from build123d import *

# Parameters (mm, degrees)
F0_W     = 80
F0_H     = 90
F1_DEPTH = 50
F2_T     = -2.5
F3_R     = 19.815
F4_DEPTH = 90.001


with BuildPart() as f1:
    # F0 (on Top) → F1 (new body)
    with BuildSketch(Plane.XY):
        Rectangle(F0_W, F0_H)
    extrude(amount=F1_DEPTH)

    # F2
    f2_openings = [f1.faces().sort_by_distance(p)[0] for p in [
        (0, 0, 50),
    ]]
    offset(amount=F2_T, openings=f2_openings)

    # F3 (on face) → F4 (cut, through all)
    with BuildSketch(Plane.XZ.offset(45)):
        with Locations((0, 25)):
            Circle(F3_R)
    extrude(amount=-F4_DEPTH, mode=Mode.SUBTRACT)


solid = f1.part
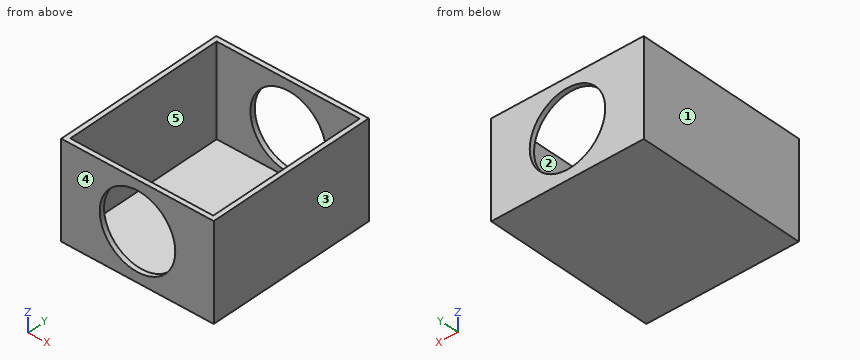
Source: CAD feature listing. Evaluate the final solid. Frame: model axes, mm. Face numbers are marked on the shaded views. A direction names the side the tool comes from. Round coordinates to 2 decimals unless told otherwise and drop trailing zeros. Loops run counter-clockwise (first coordinate to the right, second up) from the corner with the lowest first, then second, coordinate; pieces in that order, holes last. Notation, with made-up numbers: M 49,0.5 L 106,0.5 A15 ccw 106,25.5 Z; hole C 43.25,18.25 d11. An arc over 180 degrees is marked long. Return JSON: item names as keys, results as strings. Group by question number.
1. Section query C-C on y = 36.5. Output: boundary loops of the cut face in (x, z), and give its area (4 significant figures).
2. Section query A-A on x = 0. Output: boundary loops of the cut face in (y, z) (3 decimals).
3. Pin query (flat end, axial travel): pin 1 (1 mm diameter, centred on x = -25, y = -7.5, fed in from +Z); pin 2 (24 mm diameter, centred on x = 0, z = 25, fed in from -Y); pin 3 (3 mm diameter, centred on x = 12.5, y = 9.5, fed in from -Z). Return the tip coordinate at first contact, or that it passes through.
4. Section query B-B on z = 25. Output: boundary loops of the cut face in (x, y) (3 decimals), and give its area (3 significant figures).
5. Section query D-D on x = -28.5. Output: boundary loops of the cut face in (y, z).
6. Material intervals for line 1 along Z through (x, y) = (0, -43) (3 decimals); line 2 along Y through (x, z) = (-23.5, 24); line 3 along X through (y, z) = (7.5, 38.5), sorted ascending. Write a range as from..to.
7. Mould query, pull axis X, two halves, no side actions, for the marked faces 1, 2 and 3. Classes: released by +X, released by -X, zero draft, split by the parting line, or undercut.
8. Reachability of the marked faces 4 and 5 from +Z, -Z, +X, -X, +Y, -Y: full face, straight path, thin tool, end or side. Return the list, or none.
Checks:
{
 "1": {"outline": "M -40,0 L 40,0 L 40,50 L 37.5,50 L 37.5,2.5 L -37.5,2.5 L -37.5,50 L -40,50 Z", "area": "437.5 mm²"},
 "2": {"outline": "M -45,0 L 45,0 L 45,5.185 L 42.5,5.185 L 42.5,2.5 L -42.5,2.5 L -42.5,5.185 L -45,5.185 Z; M -45,44.815 L -42.5,44.815 L -42.5,50 L -45,50 Z; M 42.5,44.815 L 45,44.815 L 45,50 L 42.5,50 Z"},
 "3": {"pin 1": "stops at z = 2.5", "pin 2": "passes through", "pin 3": "stops at z = 0"},
 "4": {"outline": "M -40,-45 L -19.815,-45 L -19.815,-42.5 L -37.5,-42.5 L -37.5,42.5 L -19.815,42.5 L -19.815,45 L -40,45 Z; M 19.815,-45 L 40,-45 L 40,45 L 19.815,45 L 19.815,42.5 L 37.5,42.5 L 37.5,-42.5 L 19.815,-42.5 Z", "area": "627 mm²"},
 "5": {"outline": "M -45,0 L 45,0 L 45,50 L 42.5,50 L 42.5,2.5 L -42.5,2.5 L -42.5,50 L -45,50 Z"},
 "6": {"line 1": "z = 0..5.185, 44.815..50", "line 2": "y = -45..-42.5, 42.5..45", "line 3": "x = -40..-37.5, 37.5..40"},
 "7": {"face 1": "released by -X", "face 2": "undercut", "face 3": "released by +X"},
 "8": {"face 4": "+Z, -Z, +X, -X, -Y", "face 5": "+Z"}
}
